Autodesk Inventor part; units mm, degrees
ref_plane "YZ Plane" through (0, 0, 0) normal (1, 0, 0) x (0, 1, 0)
ref_plane "XZ Plane" through (0, 0, 0) normal (0, 1, 0) x (-1, 0, 0)
ref_plane "XY Plane" through (0, 0, 0) normal (0, 0, 1) x (1, 0, 0)
sketch "Sketch1" plane through (0, 0, 0) normal (0, 1, 0) x (-1, 0, 0)
  circle A0 centre (0, 0) radius 3.993
  circle A1 centre (0, 0) radius 2.0625
  dimension "d0" = 7.986
  dimension "d1" = 4.125
extrude "Extrusion1" add sketch "Sketch1" along normal blind 6
sketch "Sketch2" plane through (0, 6, 0) normal (0, 1, 0) x (1, 0, 0)
  circle A0 centre (0, 0) radius 2.0625
  circle A1 centre (0, 0) radius 3.993
  circle A2 centre (0, 0) radius 6
  dimension "d4" = 12
extrude "Extrusion2" add sketch "Sketch2" along normal blind 1 contours A1 | A2
sketch "Sketch3" plane through (0, 0, 0) normal (0, -1, 0) x (1, 0, 0)
  circle A0 centre (0, 0) radius 2
  circle A1 centre (0, 0) radius 2.2361
  dimension "d7" = 4
extrude "Extrusion3" add sketch "Sketch3" against normal blind 7
properties part number "eje de rodaje"
Here's how the part is built. I have some questions about the finished solid (model axes, mm). A direction names the side the tool comes from. Coordinates: 2 decimals unless noted, no trailing zeros. Loops run counter-clockwise (first coordinate to the right, second up) from the corner with the lowest first, then second, coordinate; pieces in that order, holes last. Notation, with made-up numbers: (50.25, 59.5) - (90.25, 59.5) arc R14 cw to (90.25, 76.5) - close; hole circle Ø5 at (46.25, 54). An arc over 180 degrees is marked (long way). Return JSON: item names as keys, results as strings. Group by question number.
Item 1: I need wall thicknesses on line 1 (Z direction, x = 0, y = 3.25); line 2 (Y direction, x = 5.25, z = -0.5); line 3 (Z direction, x = -1.75, y = 1.5). Which ranges of each line are inside material? Lowest first, please. Write a range as from..to.
Item 2: On a 3-axis mill with a long thin cutter (end or side, diameter ignored), from which of +Z, -Z, +X, -X, +Y, -Y can I reach the whole of each face in a straight line? I mean faces 4 (the face through (-1.4, 6, 3.9)), 5 (the face through (2, 0, -1)). Say none if no direction works.
Item 3: We'd pull the mould along X, two halves only. Please class faces 1 (the face through (0, 3, -2)), 2 (the face through (0.866, 2.958, 3.898)), 3 (the face through (3, 7, 0)): +X half, -X half, draft (parallel to the pull), parting line (faces both ways), or undercut.
Item 4: If we section it at C-C on y = 2.75: Write out the boundary of the cut face in (x, z), and give its area (3 significant figures).
Item 5: Will these pins go through, and if not, where does the flat tip stop? P1, Ø4, axis at y = 0.5, z = 3.5, coming from the -X side; P2, Ø1, axis at y = 6, z = 4.5, coming from the +X side; P3, Ø4, axis at x = -4.5, y = 4.5, coming from the +Z side.
Item 6: If we section it at D-D on z = -3.5: Write out the boundary of the cut face in (x, y), and give its area (3 significant figures).
Item 7: If we section it at A-A on x = 0: Write out the boundary of the cut face in (y, z), and give its area (3 significant figures).
Item 8: If we section it at B-B on z = 0: Write out the boundary of the cut face in (x, y), and give its area (3 significant figures).
Calculated:
{
 "1": {"line 1": "z = -3.99..-2, 2..3.99", "line 2": "y = 6..7", "line 3": "z = -3.59..-0.97, 0.97..3.59"},
 "2": {"face 4": "-Y", "face 5": "+Z, -Z, +X, -X, -Y"},
 "3": {"face 1": "undercut", "face 2": "parting line", "face 3": "draft"},
 "4": {"outline": "circle Ø7.99 at (0, 0); hole circle Ø4 at (0, 0)", "area": "37.5 mm^2"},
 "5": {"P1": "stops at x = -3.7", "P2": "stops at x = 4.47", "P3": "stops at z = 5.09"},
 "6": {"outline": "(-4.87, 6) - (-1.92, 6) - (-1.92, 0) - (1.92, 0) - (1.92, 6) - (4.87, 6) - (4.87, 7) - (-4.87, 7) - close", "area": "32.8 mm^2"},
 "7": {"outline": "(0, -3.99) - (6, -3.99) - (6, -6) - (7, -6) - (7, -2) - (0, -2) - close; (0, 2) - (7, 2) - (7, 6) - (6, 6) - (6, 3.99) - (0, 3.99) - close", "area": "31.9 mm^2"},
 "8": {"outline": "(-6, 6) - (-3.99, 6) - (-3.99, 0) - (-2, 0) - (-2, 7) - (-6, 7) - close; (2, 0) - (3.99, 0) - (3.99, 6) - (6, 6) - (6, 7) - (2, 7) - close", "area": "31.9 mm^2"}
}
